```python
from build123d import *

# Parameters (mm, degrees)
SKETCH2_R           = 30
BOSS_EXTRUDE1_DEPTH = 2
SKETCH3_W           = 64
SKETCH3_H           = 64
BOSS_EXTRUDE2_DEPTH = 68
FILLET1_R           = 8
BOSS_EXTRUDE3_START = -8
SKETCH4_R           = 32
BOSS_EXTRUDE3_DEPTH = 21
FILLET2_R           = 4
SKETCH5_R           = 6
BOSS_EXTRUDE4_DEPTH = 12
SKETCH6_R           = 24
BOSS_EXTRUDE5_DEPTH = 2
SKETCH7_R           = 26
SKETCH8_R           = 23
CUT_EXTRUDE1_DEPTH  = 26
SKETCH13_R          = 26
CUT_EXTRUDE2_DEPTH  = 26
CUT_EXTRUDE3_REACH  = 206.397
SKETCH14_R          = 18
SKETCH15_R          = 24
CUT_EXTRUDE4_DEPTH  = 4
SKETCH20_R          = 28
CUT_EXTRUDE5_DEPTH  = 2.5
FILLET3_R           = 2
SKETCH26_R          = 6
CUT_EXTRUDE6_DEPTH  = 170.49926259


with BuildPart() as part:
    # Sketch1 → Revolve1 (revolve)
    with BuildSketch(Plane.XY, mode=Mode.PRIVATE) as revolve1_sk:
        with BuildLine():
            Line((0, 0), (50, 0))
            Line((50, 0), (50, 12))
            Line((50, 12), (26, 12))
            Line((26, 12), (20, 28))
            ThreePointArc((20, 28), (28.844410204, 39.123585533), (32, 52.979991994))
            Line((32, 52.979991994), (32, 133))
            Line((32, 133), (0, 133))
            Line((0, 133), (0, 0))
        make_face()
    revolve(revolve1_sk.sketch.rotate(Axis((0, 133, 0), (0, -1, 0)), 90), axis=Axis((0, 133, 0), (0, -1, 0)))

    # Sketch2 → Boss-Extrude1 (add)
    with BuildSketch(Plane.XZ):
        with Locations(Location((0, 0, 0), (0, 0, 270))):
            Circle(SKETCH2_R)
    extrude(amount=BOSS_EXTRUDE1_DEPTH)

    # Sketch3 → Boss-Extrude2 (add)
    with BuildSketch(Plane(origin=(0, 0, 0), x_dir=(0, 0, -1), z_dir=(1, 0, 0))):
        with Locations((0, 86)):
            Rectangle(SKETCH3_W, SKETCH3_H)
    extrude(amount=BOSS_EXTRUDE2_DEPTH)

    # Fillet1
    # the kernel refuses this fillet: 8 mm, written as the material it takes off along each edge
    with BuildSketch(Plane(origin=(60, 110, 24), x_dir=(0, 1, 0), z_dir=(0, 0, 1))) as fillet1_piece_1_section:
        Polygon((0, 0), (FILLET1_R * 1.02, 0), (FILLET1_R * 1.02, -FILLET1_R * 1.02), (0, -FILLET1_R * 1.02), align=None)
    fillet1_piece_1 = extrude(amount=FILLET1_R * 1.02, mode=Mode.PRIVATE)
    fillet1_piece_1 = fillet1_piece_1 - Plane(origin=(60, 110, 24), x_dir=(-0.7071067811865475, -0.7071067811865475, 0), z_dir=(0, 0, 1)) * Sphere(FILLET1_R, mode=Mode.PRIVATE)
    add(fillet1_piece_1, mode=Mode.SUBTRACT)
    with BuildSketch(Plane(origin=(60, 62, 24), x_dir=(0, -1, 0), z_dir=(0, 0, 1))) as fillet1_piece_2_section:
        Polygon((0, 0), (FILLET1_R * 1.02, 0), (FILLET1_R * 1.02, FILLET1_R * 1.02), (0, FILLET1_R * 1.02), align=None)
    fillet1_piece_2 = extrude(amount=FILLET1_R * 1.02, mode=Mode.PRIVATE)
    fillet1_piece_2 = fillet1_piece_2 - Plane(origin=(60, 62, 24), x_dir=(-0.7071067811865475, 0.7071067811865475, 0), z_dir=(0, 0, 1)) * Sphere(FILLET1_R, mode=Mode.PRIVATE)
    add(fillet1_piece_2, mode=Mode.SUBTRACT)
    with BuildSketch(Plane(origin=(60, 62, -24), x_dir=(0, -1, 0), z_dir=(0, 0, -1))) as fillet1_piece_3_section:
        Polygon((0, 0), (FILLET1_R * 1.02, 0), (FILLET1_R * 1.02, -FILLET1_R * 1.02), (0, -FILLET1_R * 1.02), align=None)
    fillet1_piece_3 = extrude(amount=FILLET1_R * 1.02, mode=Mode.PRIVATE)
    fillet1_piece_3 = fillet1_piece_3 - Plane(origin=(60, 62, -24), x_dir=(-0.7071067811865475, 0.7071067811865475, 0), z_dir=(0, 0, -1)) * Sphere(FILLET1_R, mode=Mode.PRIVATE)
    add(fillet1_piece_3, mode=Mode.SUBTRACT)
    with BuildSketch(Plane(origin=(60, 110, -24), x_dir=(0, 0, -1), z_dir=(0, 1, 0))) as fillet1_piece_4_section:
        Polygon((0, 0), (FILLET1_R * 1.02, 0), (FILLET1_R * 1.02, -FILLET1_R * 1.02), (0, -FILLET1_R * 1.02), align=None)
    fillet1_piece_4 = extrude(amount=FILLET1_R * 1.02, mode=Mode.PRIVATE)
    fillet1_piece_4 = fillet1_piece_4 - Plane(origin=(60, 110, -24), x_dir=(-0.7071067811865475, 0, 0.7071067811865475), z_dir=(0, 1, 0)) * Sphere(FILLET1_R, mode=Mode.PRIVATE)
    add(fillet1_piece_4, mode=Mode.SUBTRACT)
    with BuildSketch(Plane(origin=(-20, 118, 32), x_dir=(0, -1, 0), z_dir=(1, 0, 0))) as fillet1_piece_5_section:
        with BuildLine():
            CenterArc((FILLET1_R, FILLET1_R), FILLET1_R, 180, 90)
            Line((0, FILLET1_R), (0, 0))
            Line((0, 0), (FILLET1_R, 0))
        make_face()
    fillet1_piece_5 = extrude(amount=80, mode=Mode.PRIVATE)
    fillet1_piece_5 = fillet1_piece_5 - Plane(origin=(0, 116.13109064, 0), x_dir=(0, 0, 1), z_dir=(0, 1, 0)) * Cylinder(32, 192, mode=Mode.PRIVATE)
    add(fillet1_piece_5, mode=Mode.SUBTRACT)
    with BuildSketch(Plane(origin=(-20, 54, 32), x_dir=(0, 1, 0), z_dir=(1, 0, 0))) as fillet1_piece_6_section:
        with BuildLine():
            CenterArc((FILLET1_R, -FILLET1_R), FILLET1_R, 90, 90)
            Line((0, -FILLET1_R), (0, 0))
            Line((0, 0), (FILLET1_R, 0))
        make_face()
    fillet1_piece_6 = extrude(amount=80, mode=Mode.PRIVATE)
    fillet1_piece_6 = fillet1_piece_6 - Plane(origin=(0, 55.86890936, 0), x_dir=(0, 0, 1), z_dir=(0, 1, 0)) * Cylinder(32, 192, mode=Mode.PRIVATE)
    add(fillet1_piece_6, mode=Mode.SUBTRACT)
    with BuildSketch(Plane(origin=(-20, 54, -32), x_dir=(0, 1, 0), z_dir=(1, 0, 0))) as fillet1_piece_7_section:
        with BuildLine():
            CenterArc((FILLET1_R, FILLET1_R), FILLET1_R, 180, 90)
            Line((0, FILLET1_R), (0, 0))
            Line((0, 0), (FILLET1_R, 0))
        make_face()
    fillet1_piece_7 = extrude(amount=80, mode=Mode.PRIVATE)
    fillet1_piece_7 = fillet1_piece_7 - Plane(origin=(0, 55.868908347, 0), x_dir=(0, 0, 1), z_dir=(0, 1, 0)) * Cylinder(32, 193, mode=Mode.PRIVATE)
    add(fillet1_piece_7, mode=Mode.SUBTRACT)
    with BuildSketch(Plane(origin=(-20, 118, -32), x_dir=(0, 0, 1), z_dir=(1, 0, 0))) as fillet1_piece_8_section:
        with BuildLine():
            CenterArc((FILLET1_R, FILLET1_R), FILLET1_R, 180, 90)
            Line((0, FILLET1_R), (0, 0))
            Line((0, 0), (FILLET1_R, 0))
        make_face()
    fillet1_piece_8 = extrude(amount=80, mode=Mode.PRIVATE)
    fillet1_piece_8 = fillet1_piece_8 - Plane(origin=(0, 116.131091799, 0), x_dir=(0, 0, 1), z_dir=(0, 1, 0)) * Cylinder(32, 192, mode=Mode.PRIVATE)
    add(fillet1_piece_8, mode=Mode.SUBTRACT)
    with BuildSketch(Plane(origin=(68, 110, 32), x_dir=(-1, 0, 0), z_dir=(0, -1, 0)), Plane(origin=(68, 54, 24), x_dir=(-1, 0, 0), z_dir=(0, 0, -1)), Plane(origin=(68, 62, -32), x_dir=(-1, 0, 0), z_dir=(0, 1, 0)), Plane(origin=(68, 118, -24), x_dir=(-1, 0, 0), z_dir=(0, 0, 1))) as fillet1_piece_9:
        with BuildLine():
            CenterArc((FILLET1_R, FILLET1_R), FILLET1_R, 180, 90)
            Line((0, FILLET1_R), (0, 0))
            Line((0, 0), (FILLET1_R, 0))
        make_face()
    extrude(amount=48, mode=Mode.SUBTRACT)

    # Sketch4 → Boss-Extrude3 (add)
    with BuildSketch(Plane.XY.offset(32).offset(BOSS_EXTRUDE3_START)):
        with Locations((36, 86)):
            Circle(SKETCH4_R)
    extrude(amount=BOSS_EXTRUDE3_DEPTH)

    # Fillet2
    fillet2_edges = [part.edges().sort_by_distance(p)[0] for p in [
        (0, 28, -20),
        (0, 12, -26),
    ]]
    fillet(fillet2_edges, radius=FILLET2_R)



with BuildPart() as body_2:
    # Sketch5 → Boss-Extrude4 (new body)
    with BuildSketch(Plane.XY.offset(-73)):
        with BuildLine():
            Line((-8.631578947, 69.266137306), (24.210526316, 56.250910766))
            ThreePointArc((24.210526316, 56.250910766), (36, 54), (47.789473684, 56.250910766))
            Line((47.789473684, 56.250910766), (80.631578947, 69.266137306))
            ThreePointArc((80.631578947, 69.266137306), (92, 86), (80.631578947, 102.733862694))
            Line((80.631578947, 102.733862694), (47.789473684, 115.749089234))
            ThreePointArc((47.789473684, 115.749089234), (36, 118), (24.210526316, 115.749089234))
            Line((24.210526316, 115.749089234), (-8.631578947, 102.733862694))
            ThreePointArc((-8.631578947, 102.733862694), (-20, 86), (-8.631578947, 69.266137306))
        make_face()
        with Locations((-2, 86)):
            Circle(SKETCH5_R, mode=Mode.SUBTRACT)
        with Locations((74, 86)):
            Circle(SKETCH5_R, mode=Mode.SUBTRACT)
    extrude(amount=BOSS_EXTRUDE4_DEPTH)

    # Sketch6 → Boss-Extrude5 (add)
    with BuildSketch(Plane(origin=(0, 0, -73), x_dir=(-1, 0, 0), z_dir=(0, 0, -1))):
        with Locations(Location((-36, 86, 0), (0, 0, 180))):
            Circle(SKETCH6_R)
    extrude(amount=BOSS_EXTRUDE5_DEPTH)


with BuildPart() as part_1:
    add(part.part)

    add(body_2.part)  # Loft2 merges body 2
    # Sketch7 → Loft2 section 0
    with BuildSketch(Plane.XY.offset(-61)):
        with Locations((36, 86)):
            Circle(SKETCH7_R)
    # Sketch8 → Loft2 section 1
    with BuildSketch(Plane(origin=(0, 0, -32), x_dir=(-1, 0, 0), z_dir=(0, 0, -1))):
        with Locations((-36, 86)):
            Circle(SKETCH8_R)
    loft()

    # Sketch11 → Cut-Extrude1 (cut, symmetric)
    with BuildSketch(Plane.XY):
        with BuildLine():
            Line((60, 112), (0, 112))
            Line((0, 112), (0, 60))
            Line((0, 60), (60, 60))
            ThreePointArc((60, 60), (61.414213562, 60.585786438), (62, 62))
            Line((62, 62), (62, 110))
            ThreePointArc((62, 110), (61.414213562, 111.414213562), (60, 112))
        make_face()
    extrude(amount=CUT_EXTRUDE1_DEPTH, both=True, mode=Mode.SUBTRACT)

    # Sketch13 → Cut-Extrude2 (cut, symmetric)
    with BuildSketch(Plane(origin=(0, 86, 0), x_dir=(-1, 0, 0), z_dir=(0, -1, 0))):
        Circle(SKETCH13_R)
    extrude(amount=CUT_EXTRUDE2_DEPTH, both=True, mode=Mode.SUBTRACT)

    # Sketch14 → Cut-Extrude3 (cut, up to next)
    with BuildSketch(Plane(origin=(0, 0, -75), x_dir=(-1, 0, 0), z_dir=(0, 0, -1)), mode=Mode.PRIVATE) as cut_extrude3_sk1:
        with Locations((-36, 86)):
            Circle(SKETCH14_R)
    cut_extrude3_tool1 = extrude(cut_extrude3_sk1.sketch, amount=-CUT_EXTRUDE3_REACH, mode=Mode.PRIVATE) & part_1.part
    add(cut_extrude3_tool1.solids().sort_by_distance((36, 86, -75))[0], mode=Mode.SUBTRACT)

    # Sketch15 → Cut-Extrude4 (cut)
    with BuildSketch(Plane.XY.offset(45)):
        with Locations((36, 86)):
            Circle(SKETCH15_R)
    extrude(amount=-CUT_EXTRUDE4_DEPTH, mode=Mode.SUBTRACT)

    # Sketch19 → M39x2.0 Tapped Hole1 (revolve, cut)
    with BuildSketch(Plane(origin=(36, 86, 41), x_dir=(0, -1, 0), z_dir=(1, 0, 0))):
        Polygon((0, 0), (0, 15), (18.5, 15), (18.5, 1.025), (19.525, 0), align=None)
    revolve(axis=Axis((36, 86, 47.35), (0, 0, -1)), mode=Mode.SUBTRACT)

    # Sketch20 → Cut-Extrude5 (cut)
    with BuildSketch(Plane(origin=(0, 133, 0), x_dir=(1, 0, 0), z_dir=(0, 1, 0))):
        with Locations(Location((0, 0, 0), (0, 0, 270))):
            Circle(SKETCH20_R)
    extrude(amount=-CUT_EXTRUDE5_DEPTH, mode=Mode.SUBTRACT)

    # Sketch22 → M48x2.0 Tapped Hole1 (revolve, cut)
    with BuildSketch(Plane(origin=(0, 130.5, 0), x_dir=(0, 0, 1), z_dir=(1, 0, 0))):
        Polygon((0, 0), (0, 18.5), (23, 18.5), (23, 1.025), (24.025, 0), align=None)
    revolve(axis=Axis((0, 136.85, 0), (0, -1, 0)), mode=Mode.SUBTRACT)

    # Sketch23 → Cut-Revolve1 (revolve, cut)
    with BuildSketch(Plane.XY, mode=Mode.PRIVATE) as cut_revolve1_sk:
        Polygon((0, 44), (18, 44), (18, 34), (12.5, 34), (12.5, -2), (0, -2), align=None)
    revolve(cut_revolve1_sk.sketch.rotate(Axis((0, -2, 0), (0, 1, 0)), 90), axis=Axis((0, -2, 0), (0, 1, 0)), mode=Mode.SUBTRACT)

    # Sketch25 → M33x2.0 Tapped Hole1 (revolve, cut)
    with BuildSketch(Plane(origin=(0, 44, 0), x_dir=(0, 0, -1), z_dir=(1, 0, 0))):
        Polygon((0, 0), (0, 16), (15.5, 16), (15.5, 1.025), (16.525, 0), align=None)
    revolve(axis=Axis((0, 37.65, 0), (0, 1, 0)), mode=Mode.SUBTRACT)

    # Fillet3
    fillet3_edges = [part_1.edges().sort_by_distance(p)[0] for p in [
        (64.210526316, 62.758524036, -61),
        (7.789473684, 109.241475964, -61),
        (-20, 86, -61),
        (10, 86, -61),
        (7.789473684, 62.758524036, -61),
        (36, 54, -61),
        (92, 86, -61),
        (64.210526316, 109.241475964, -61),
        (36, 118, -61),
        (30, 112, 26),
        (61.414213562, 111.414213562, 26),
        (62, 86, 26),
        (61.414213562, 60.585786438, 26),
        (30, 60, 26),
        (30, 60, -26),
        (61.414213562, 60.585786438, -26),
        (62, 86, -26),
        (61.414213562, 111.414213562, -26),
        (30, 112, -26),
        (-26, 112, 0),
        (-26, 60, 0),
        (0, 133, -32),
        (0, 12, -50),
    ]]
    fillet(fillet3_edges, radius=FILLET3_R)

    # Sketch26 → Cut-Extrude6 (cut, through all)
    with BuildSketch(Plane(origin=(0, 12, 0), x_dir=(1, 0, 0), z_dir=(0, 1, 0))):
        with Locations(Location((0, 37.5, 0), (0, 0, 270))):
            Circle(SKETCH26_R)
        with Locations(Location((37.5, 0, 0), (0, 0, 270))):
            Circle(SKETCH26_R)
        with Locations(Location((0, -37.5, 0), (0, 0, 270))):
            Circle(SKETCH26_R)
        with Locations(Location((-37.5, 0, 0), (0, 0, 270))):
            Circle(SKETCH26_R)
    extrude(amount=-CUT_EXTRUDE6_DEPTH, mode=Mode.SUBTRACT)

    # Split1
    split(bisect_by=Plane.XY, keep=Keep.TOP)


solid = part_1.part
```
Verification items for the finished model (mm, model axes). A direction names the side the tool comes from. Give positions to 0.01 mm unless a question says otherwise; leave off trailing zeros. Order: outer loops, then holes, each group sorted by start corner. A loop starts at its lowest first (then second) coordinate and runs counter-clockwise, first axis right, second up. Notation, with made-up numbers: M -23.75,30.25 L -16.75,30.25 A12 cw -16.75,34.25 Z; hole C 21.5,12 d4. An arc over 180 degrees is marked long. Answer in a Markdown table with one row per item. Add a question column.
Item 1: Mould release check, pull along Y, two halves, no side actions. Record for faces 1 (the flat face through (0, -2, 15)), 2 (the flat face through (59, 63, 32)), 3 (the conical face through (0.485, 22.477, 22.066)): released by +Y, released by -Y, zero draft, split by the parting line, or undercut.
Item 2: Section check A-A, the plane z = 37.5. State how many separate pieces and enclosed holes the cut face has, and give its area (3 significant figures).
Item 3: Gauge pin test, flat ends, axial feed: pin 1 (24 mm diameter, centred on x = 20.5, y = 89, fed in from -Z); pin 2 (2 mm diameter, centred on x = -26.5, z = 28, fed in from +Y); pin 3 (9 mm diameter, centred on x = 8, z = 5, fed in from +Y). Record the tip position at first contact, or that the pin passes through.
Item 4: Scan lines: probe 1 along Y at (x, z) = (31.5, 15); probe 2 along Y at (x, z) = (36, 41.8); probe 3 along Y at (x, z) = (36, 37). Record each from-to range of solid material in increasing order. Write a range as from..to.
Item 5: Tool access check on faces 4 (the flat face through (0.1, 130.5, 24.3)), 5 (the cylindrical face through (-18.18, 85.66, 18.59)), 6 (the flat face through (45, 54, 12)), 7 (the cylindrical face through (19.249, 56.364, 29.678)), 8 (the flat face through (-1, 0, 31)). Record the directions out of +Z, -Z, +X, -X, +Y, -Y that give a thin tool (end or side, any length) a straight path to the whole face; none if there is none.
Item 6: Section check C-C, the plane y = 42.5. Enter the section's corners in (x, z), and give its area (3 significant figures).
Filled sheet:
| question | item | result |
|---|---|---|
| 1 | face 1 | released by -Y |
| 1 | face 2 | zero draft |
| 1 | face 3 | undercut |
| 2 | separate pieces | 3 |
| 2 | enclosed holes | 1 |
| 2 | area | 2,790 mm^2 |
| 3 | pin 1 | stops at z = 26 |
| 3 | pin 2 | stops at y = 12 |
| 3 | pin 3 | stops at y = 34 |
| 4 | probe 1 | y = 0..12, 54..60, 112..118 |
| 4 | probe 2 | y = 54..62, 110..118 |
| 4 | probe 3 | y = 54..67.5, 104.5..118 |
| 5 | face 4 | -Z, +Y |
| 5 | face 5 | -Z |
| 5 | face 6 | +Z, +X |
| 5 | face 7 | +Z |
| 5 | face 8 | +Z, -Y |
| 6 | outline | M -30.24,0 L -18,0 A18 cw 18,0 L 30.24,0 A30.24 ccw Z |
| 6 | area | 927 mm^2 |
